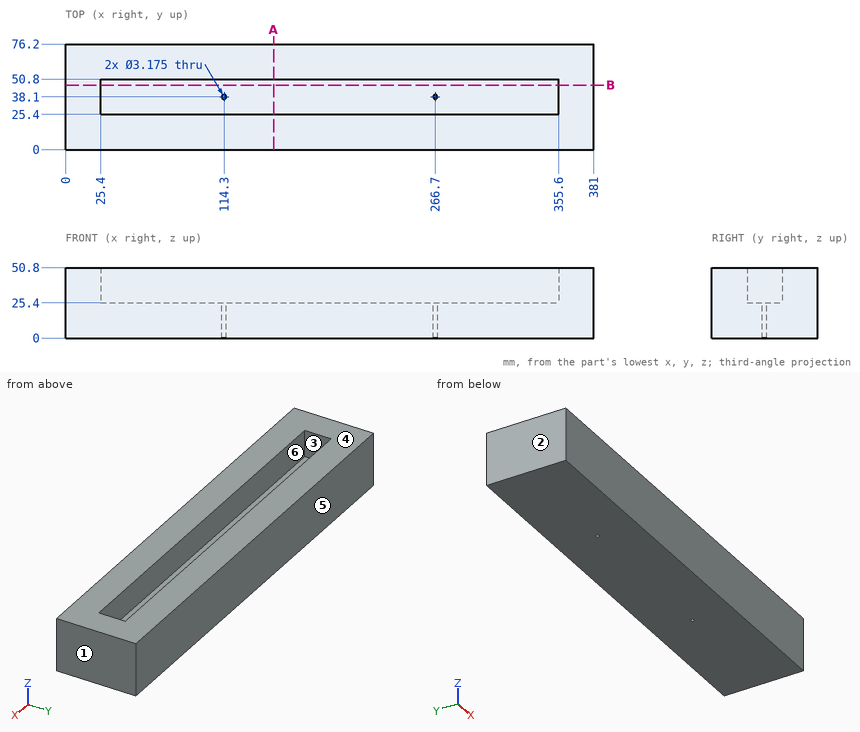
Drawing for the job (mm, zero at the part's lowest x, y, z). A direction names the side the tool comes from. Coordinates: 2 decimals unless noted, no trailing zeros. Order: outer loops, then holes, each group sorted by start corner. A loop starts at its lowest first (then second) coordinate and runs counter-clockwise, first axis right, second up.
Item 1: 3-axis set-ups, long thin cutter, end or side, ignore diameter. For the marked faces 5 and 6: which of +Z, -Z, +X, -X, +Y, -Y reach the whole face in a straight line?
Check sheet entries:
face 5: +Z, -Z, +X, -X, +Y
face 6: +Z
Item 2: Band-saw the part on B-B on y = 46.5. List the corners of the cut face in (x, z), plus the area to 3 significant figures.
Check sheet entries:
outline: (0, 0) - (381, 0) - (381, 50.8) - (355.6, 50.8) - (355.6, 25.4) - (25.4, 25.4) - (25.4, 50.8) - (0, 50.8) - close
area: 11,000 mm2
Item 3: Two-plate mould, pull along X, no slides. Class the marked faces 1, 2, 3 and 4: +X half, -X half, draft (parallel to the pull), parting line (faces both ways), or undercut.
Check sheet entries:
face 1: +X half
face 2: -X half
face 3: undercut
face 4: draft
Item 4: Band-saw the part on A-A on x = 150. List the corners of the cut face in (y, z).
Check sheet entries:
outline: (0, 0) - (76.2, 0) - (76.2, 50.8) - (50.8, 50.8) - (50.8, 25.4) - (25.4, 25.4) - (25.4, 50.8) - (0, 50.8) - close
Item 5: Pin check, flat tip, straight feed: pin 1 Ø10 at (x, y) = (102, 41) entering from +Z. Stop position of the tip, or through.
Check sheet entries:
pin 1: stops at z = 25.4
Item 6: Drill centre lines: L1, parallel to X at y = 38.1, z = 9.25; L2, parallel to Y at x = 266.7, z = 5.75; L3, parallel to X at y = 38, z = 39. Where is each one in solid material? Low to high.
Check sheet entries:
L1: x = 0 to 112.71, 115.89 to 265.11, 268.29 to 381
L2: y = 0 to 36.51, 39.69 to 76.2
L3: x = 0 to 25.4, 355.6 to 381
